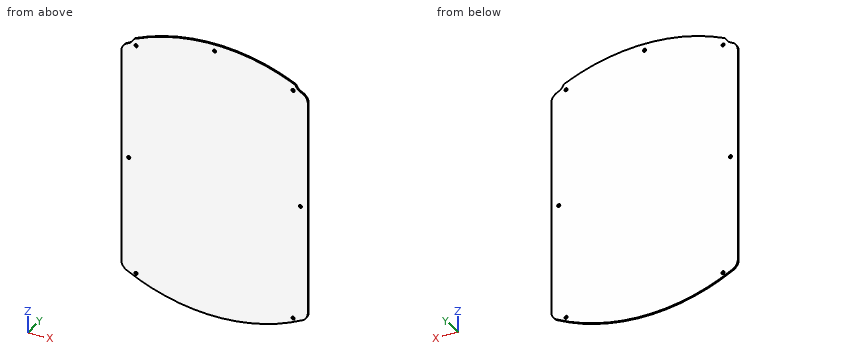
from build123d import *

# Parameters (mm, degrees)
BASE_FLANGE1_DEPTH = 1.5
TAB1_DEPTH         = 1.5
FILLET1_R          = 10
FILLET2_R          = 5
SKETCH9_R          = 1.6
CUT_EXTRUDE1_DEPTH = 172.686487668


# Sheet-metal steps are written as plain solids
with BuildPart() as part:
    # Base-Flange1: sheet metal written as solids
    # Sketch1 → Base-Flange1 (new body)
    with BuildSketch(Plane(origin=(0, 0, 0), x_dir=(1, 0, 0), z_dir=(0, 1, 0))):
        with BuildLine():
            Line((95, -115), (95, 115))
            ThreePointArc((95, 115), (0, 140), (-95, 115))
            Line((-95, 115), (-95, -115))
            ThreePointArc((-95, -115), (0, -140), (95, -115))
        make_face()
    extrude(amount=-BASE_FLANGE1_DEPTH)

    # Tab1: sheet metal written as solids
    # Sketch2 → Tab1 (add)
    with BuildSketch(Plane(origin=(0, 0, 0), x_dir=(1, 0, 0), z_dir=(0, 1, 0))):
        with BuildLine():
            Line((-82.5, -124.791310249), (-82.5, -121.478508705))
            ThreePointArc((-82.5, -121.478508705), (0, -140), (82.5, -121.478508705))
            Line((82.5, -121.478508705), (82.5, -124.791310249))
            ThreePointArc((82.5, -124.791310249), (0, -143), (-82.5, -124.791310249))
        make_face()
    extrude(amount=-TAB1_DEPTH)

    # Fillet1
    # the kernel refuses this fillet: 10 mm, written as the material it adds along each edge
    with BuildSketch(Plane(origin=(-82.5, 0, 121.478508705), x_dir=(-0.8978334247322157, 0, -0.4403352602661074), z_dir=(0, -1, 0))) as fillet1_piece_1:
        with BuildLine():
            CenterArc((5.658454261, -9.998979067), FILLET1_R, 90.818728741, 44.556283737)
            Line((-1.45874333, -2.974343955), (0, 0))
            ThreePointArc((0, 0), (2.757782001, -0.019704015), (5.515564002, 0))
        make_face()
    extrude(amount=1.5)
    with BuildSketch(Plane(origin=(82.5, 0, 121.478508705), x_dir=(0.8978334247322127, 0, -0.44033526026611364), z_dir=(0, -1, 0))) as fillet1_piece_2:
        with BuildLine():
            CenterArc((5.658454261, 9.998979067), FILLET1_R, 224.624987522, 44.556283737)
            Line((-1.45874333, 2.974343955), (0, 0))
            ThreePointArc((0, 0), (2.757782001, 0.019704015), (5.515564002, 0))
        make_face()
    extrude(amount=1.5)
    # the kernel refuses this fillet: 10 mm, written as the material it takes off along each edge
    with BuildSketch(Plane(origin=(-95, 15.245934007, 115), x_dir=(0, 0, -1), z_dir=(0, -1, 0))) as fillet1_2_piece_1:
        with BuildLine():
            CenterArc((5.938283361, 10), FILLET1_R, 207.676630301, 62.323369699)
            ThreePointArc((-2.917548149, 5.355191257), (-1.479926921, 2.6660714), (0, 0))
            Line((0, 0), (5.938283361, 0))
        make_face()
    extrude(amount=31.991868015, mode=Mode.SUBTRACT)
    with BuildSketch(Plane(origin=(95, 15.245934007, 115), x_dir=(0, 0, -1), z_dir=(0, -1, 0)), Plane(origin=(-95, 15.245934007, -115), x_dir=(0, 0, 1), z_dir=(0, -1, 0))) as fillet1_2_piece_2:
        with BuildLine():
            CenterArc((5.938283361, -10), FILLET1_R, 90, 62.323369699)
            ThreePointArc((-2.917548149, -5.355191257), (-1.479926921, -2.6660714), (0, 0))
            Line((0, 0), (5.938283361, 0))
        make_face()
    extrude(amount=31.991868015, mode=Mode.SUBTRACT)
    with BuildSketch(Plane(origin=(95, 15.245934007, -115), x_dir=(-0.8781343363797829, 0, -0.47841413782500014), z_dir=(0, -1, 0))) as fillet1_2_piece_3:
        with BuildLine():
            CenterArc((5.94038465, -9.998751897), FILLET1_R, 89.094752314, 62.323369699)
            Line((-2.840958714, -5.214610518), (0, 0))
            ThreePointArc((0, 0), (3.049186801, 0.024088395), (6.098373603, 0))
        make_face()
    extrude(amount=31.991868015, mode=Mode.SUBTRACT)

    # Fillet2
    fillet2_edges = [part.edges().sort_by_distance(p)[0] for p in [
        (82.5, -0.75, 124.791310249),
        (-82.5, -0.75, 124.791310249),
    ]]
    fillet(fillet2_edges, radius=FILLET2_R)

    # Sketch9 → Cut-Extrude1 (cut, through all)
    with BuildSketch(Plane(origin=(0, 0, 0), x_dir=(1, 0, 0), z_dir=(0, 1, 0))):
        with Locations(Location((-79.980506034, 118.518748697, 0), (0, 0, 270))):
            Circle(SKETCH9_R)
        with Locations(Location((79.980506034, 118.518748697, 0), (0, 0, 270))):
            Circle(SKETCH9_R)
        with Locations(Location((-79.980506034, -118.518748697, 0), (0, 0, 270))):
            Circle(SKETCH9_R)
        with Locations(Location((0, -136.25, 0), (0, 0, 270))):
            Circle(SKETCH9_R)
        with Locations(Location((79.980506034, -118.518748697, 0), (0, 0, 270))):
            Circle(SKETCH9_R)
        with Locations(Location((87.5, 0, 0), (0, 0, 270))):
            Circle(SKETCH9_R)
        with Locations(Location((-87.5, 0, 0), (0, 0, 270))):
            Circle(SKETCH9_R)
    extrude(amount=-CUT_EXTRUDE1_DEPTH, mode=Mode.SUBTRACT)


solid = part.part
Build history of the part. All positions in model axes, mm. Give positions to 0.01 mm unless a question says otherwise; leave off trailing zeros. Order: outer loops, then holes, each group sorted by start corner. A loop starts at its lowest first (then second) coordinate and runs counter-clockwise, first axis right, second up. Notation, with made-up numbers: M 71,71 L 92,71 A25 ccw 92,83 Z; hole C -19.75,47 d3. An arc over 180 degrees is marked long. Put each result on its own line as item: value.
Item 1: Slice it at A-A, the plane x = -36. Write the cut outline in (y, z).
From the geometry:
outline: M -1.5,-136.61 L 0,-136.61 L 0,139.67 L -1.5,139.67 Z
Item 2: Probe line 1 (X direction, y = -0.8, z = 0); line 2 (X direction, y = -1.05, z = 109.5); line 3 (Z direction, x = -2, y = -0.5). List the from-to ranges inside material, lowest first. Write a range as [from, to].
From the geometry:
line 1: x = [-95, -89.1], [-85.9, 85.9], [89.1, 95]
line 2: x = [-94.99, 94.99]
line 3: z = [-139.99, 142.99]
Item 3: Slice it at C-C, the plane x = -69.5. Write the cut outline in (y, z).
From the geometry:
outline: M -1.5,-127.05 L 0,-127.05 L 0,130.26 L -1.5,130.26 Z
Item 4: Slice it at B-B, the plane y = -1.1. Give the number of separate pieces and of enclosed holes in the cut face, plus the area to 3 significant figures.
From the geometry:
separate pieces: 1
enclosed holes: 7
area: 50,600 mm2
Item 5: Flat gauge pin, fed straight in: pin 1 Ø1.9 at (x, z) = (0, 136.25) entering from -Y. Where does the tip first touch, or does it go through?
From the geometry:
pin 1: passes through
